The model under review builds one solid part; all positions refer to its coordinate system, in mm. Face numbers are marked on the shaded views. A direction names the side the tool comes from. Round coordinates to 2 decimals unless told otherwise and drop trailing zeros. Write each loop counter-clockwise with the first axis right and the second up, starting at its lowest first coordinate (ties: lowest second). Pieces come first, ordered by that corner, then holes. Notation, with made-up numbers: (72.5, 60.5) -> (130.5, 60.5) arc R18 cw to (130.5, 70.5) -> close; hole circle Ø7 at (40, 43.25). An arc over 180 degrees is marked (long way). Answer as a JSON object with one key per item and string values. Group by question number.
1) Mouldability with a two-part tool opening along X and no side actions: class the marked faces 3, 4 and 5 as pulls with the +X half, pulls with the -X half, needs draft (parallel to the pull), parting line crosses it, or undercut.
2) Machinability: for the marked faces 1 and 2, which of the approach directions +Z, -Z, +X, -X, +Y, -Y give a long, thin tool a straight path to every point of the face, cutting with its end or side? Answer none if there is none.
3) Insertion check: pin 1 Ø1.5 at (x, z) = (-0.5, 3.5) entering from +Y. The pin has a flat end and moves straight along its axis. Give the tip position at first contact, or say it passes through.
4) We need section B-B, the plane x = 14.5. Write out the cut boundary in (y, z), then the cut area to 3 significant figures.
5) We need section A-A, the plane y = 2. Write out the cut boundary in (x, z), then the cut area to 3 significant figures.
6) We need section C-C, the plane z = -1.75. Write out the cut boundary in (x, y).
7) We need section D-D, the plane x = 2.5. Write out the cut boundary in (y, z), then the cut area to 3 significant figures.
8) To check wall thickness, follow probe 1 along X at (y, z) = (8, 8); probe 2 along Z at (x, y) = (15.25, 9.25); probe 3 along X at (y, z) = (7.25, 9). State the ranges of each line that lie inside material, in increasing order. Write a range as [from, to].
from build123d import *

# Parameters (mm, degrees)
SKETCH2_W             = 46.5
SKETCH2_H             = 26
BOSS_EXTRUDE1_DEPTH   = 14
CUT_EXTRUDE1_DEPTH    = 40.354955215
FILLET1_R             = 5
FILLET2_R             = 1
F_6_0MM_DOWEL_HOLE1_D = 6


with BuildPart() as part:
    # Sketch2 → Boss-Extrude1 (new body)
    with BuildSketch(Plane(origin=(0, 0, 0), x_dir=(1, 0, 0), z_dir=(0, 1, 0))):
        Rectangle(SKETCH2_W, SKETCH2_H)
    extrude(amount=BOSS_EXTRUDE1_DEPTH)

    # Sketch5 → Cut-Extrude1 (cut, through all)
    with BuildSketch(Plane.XY.offset(15.5)):
        Polygon((-8.25, 14), (-7.848214286, 9.5), (7.848214286, 9.5), (8.25, 14), align=None)
    extrude(amount=-CUT_EXTRUDE1_DEPTH, mode=Mode.SUBTRACT)

    # Fillet1
    fillet1_edges = [part.edges().sort_by_distance(p)[0] for p in [
        (-23.25, 7, -13),
        (23.25, 7, -13),
        (23.25, 7, 13),
        (-23.25, 7, 13),
    ]]
    fillet(fillet1_edges, radius=FILLET1_R)

    # Fillet2
    fillet2_edges = [part.edges().sort_by_distance(p)[0] for p in [
        (13.25, 14, 13),
        (-13.25, 14, -13),
        (-8.25, 14, 0),
        (7.848214286, 9.5, 0),
        (0, 9.5, 13),
        (0, 9.5, -13),
        (-7.848214286, 9.5, 0),
        (-8.049107143, 11.75, 13),
        (-8.049107143, 11.75, -13),
        (8.25, 14, 0),
        (8.049107143, 11.75, 13),
        (8.049107143, 11.75, -13),
        (13.25, 14, -13),
        (23.25, 14, 0),
        (21.785533906, 14, 11.535533906),
        (21.785533906, 14, -11.535533906),
        (-13.25, 14, 13),
        (-23.25, 14, 0),
        (-21.785533906, 14, 11.535533906),
        (-21.785533906, 14, -11.535533906),
    ]]
    fillet(fillet2_edges, radius=FILLET2_R)

    # Ø6.0mm Dowel Hole1 (through all)
    with Locations(Plane(origin=(0, 14, 0), x_dir=(1, 0, 0), z_dir=(0, 1, 0))):
        with Locations((15.25, 8), (15.25, -8), (-15.75, -8), (-15.75, 8)):
            Hole(F_6_0MM_DOWEL_HOLE1_D / 2)


solid = part.part
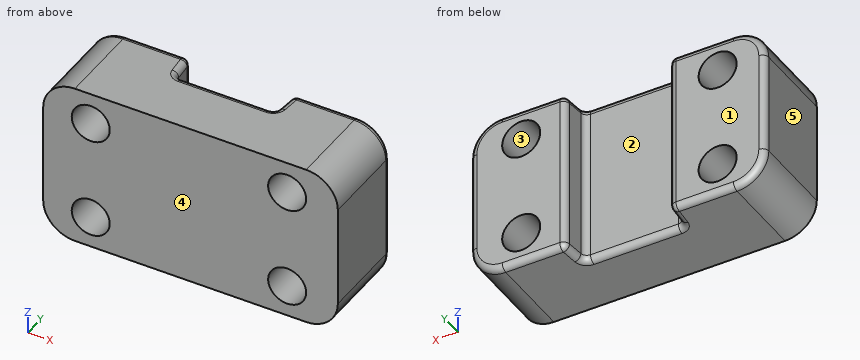
Here are the results:
{
 "1": {"face 3": "undercut", "face 4": "needs draft", "face 5": "pulls with the -X half"},
 "2": {"face 1": "+Z, -Z, +X, -X, +Y", "face 2": "+Z, -Z, +Y"},
 "3": {"pin 1": "stops at y = 9.5"},
 "4": {"outline": "(0, -13) -> (13, -13) arc R1 ccw to (14, -12) -> (14, -10.9) -> (0, -10.9) -> close; (0, -5.1) -> (14, -5.1) -> (14, 5.1) -> (0, 5.1) -> close; (0, 10.9) -> (14, 10.9) -> (14, 12) arc R1 ccw to (13, 13) -> (0, 13) -> close", "area": "201 mm^2"},
 "5": {"outline": "(-23.25, -8) arc R5 ccw to (-18.25, -13) -> (18.25, -13) arc R5 ccw to (23.25, -8) -> (23.25, 8) arc R5 ccw to (18.25, 13) -> (-18.25, 13) arc R5 ccw to (-23.25, 8) -> close; hole circle Ø6 at (-15.75, -8); hole circle Ø6 at (-15.75, 8); hole circle Ø6 at (15.25, -8); hole circle Ø6 at (15.25, 8)", "area": "1,070 mm^2"},
 "6": {"outline": "(-23.25, 0) -> (23.25, 0) -> (23.25, 13) arc R1 ccw to (22.25, 14) -> (9.16, 14) arc R1 ccw to (8.17, 13.09) -> (7.93, 10.41) arc R1 cw to (6.93, 9.5) -> (-6.93, 9.5) arc R1 cw to (-7.93, 10.41) -> (-8.17, 13.09) arc R1 ccw to (-9.16, 14) -> (-22.25, 14) arc R1 ccw to (-23.25, 13) -> close"},
 "7": {"outline": "(0, -13) -> (8.5, -13) arc R1 ccw to (9.5, -12) -> (9.5, 12) arc R1 ccw to (8.5, 13) -> (0, 13) -> close", "area": "247 mm^2"},
 "8": {"probe 1": "x = [-23.25, -18.75], [-12.75, 12.25], [18.25, 23.25]", "probe 2": "z = [-13, -11], [-5, 5], [11, 13]", "probe 3": "x = [-23.15, -18.58], [-12.92, 12.42], [18.08, 23.15]"}
}
